Geometry: final body of the model. Coordinates: model frame, mm. A direction names the side the tool comes from. Coordinates: 2 decimals unless noted, no trailing zeros. Order: outer loops, then holes, each group sorted by start corner. A loop starts at its lowest first (then second) coordinate and runs counter-clockwise, first axis right, second up. Notation, with made-up numbers: (22, -10.75) - (73, -10.75) arc R9 cw to (73, -5.75) - close; hole circle Ø2 at (62, 18). An arc over 180 degrees is marked (long way). Use one line per item in the form item = value. Start each with the question number.
```python
from build123d import *

# Parameters (mm, degrees)
CROQUIS1_R              = 1
SALIENTE_EXTRUIR1_DEPTH = 1.6
CROQUIS2_R              = 1
CORTAR_EXTRUIR1_DEPTH   = 10
CROQUIS3_R              = 6
CROQUIS3_W              = 4.6
CROQUIS3_H              = 10
CROQUIS3_W_2            = 6.6
CROQUIS3_H_2            = 6.6
CROQUIS3_W_3            = 5
CROQUIS3_H_3            = 11
CROQUIS3_H_4            = 5
SALIENTE_EXTRUIR2_DEPTH = 2
CROQUIS4_R              = 6
SALIENTE_EXTRUIR3_DEPTH = 4.5
CROQUIS5_W              = 4.6
CROQUIS5_H              = 10
SALIENTE_EXTRUIR4_DEPTH = 1.5
CROQUIS7_R              = 1.122052982
SALIENTE_EXTRUIR5_DEPTH = 1.6
CROQUIS9_R              = 1.125
CORTAR_EXTRUIR2_DEPTH   = 33.479147156


with BuildPart() as part:
    # Croquis1 → Saliente-Extruir1 (new body)
    with BuildSketch(Plane(origin=(0, 0, 0), x_dir=(1, 0, 0), z_dir=(0, 1, 0))):
        Polygon((-18.05, 13.85), (18.05, 13.85), (18.05, 10.8), (28.65, 10.8), (28.65, -10.8), (18.05, -10.8), (18.05, -13.85), (-18.05, -13.85), align=None)
        with Locations(Location((-10.35, -12.3, 0), (0, 0, 270))):
            Circle(CROQUIS1_R, mode=Mode.SUBTRACT)
        with Locations(Location((16.05, -12.3, 0), (0, 0, 270))):
            Circle(CROQUIS1_R, mode=Mode.SUBTRACT)
        with Locations(Location((16.05, 12.3, 0), (0, 0, 270))):
            Circle(CROQUIS1_R, mode=Mode.SUBTRACT)
        with Locations(Location((-10.35, 12.3, 0), (0, 0, 270))):
            Circle(CROQUIS1_R, mode=Mode.SUBTRACT)
    extrude(amount=SALIENTE_EXTRUIR1_DEPTH)

    # Croquis2 → Cortar-Extruir1 (cut)
    with BuildSketch(Plane(origin=(0, 1.6, 0), x_dir=(1, 0, 0), z_dir=(0, 1, 0))):
        with Locations(Location((24.25, 7.25, 0), (0, 0, 270))):
            Circle(CROQUIS2_R)
        with Locations(Location((24.25, -7.25, 0), (0, 0, 270))):
            Circle(CROQUIS2_R)
    extrude(amount=-CORTAR_EXTRUIR1_DEPTH, mode=Mode.SUBTRACT)

    # Croquis3 → Saliente-Extruir2 (add)
    with BuildSketch(Plane(origin=(0, 1.6, 0), x_dir=(1, 0, 0), z_dir=(0, 1, 0))):
        with Locations(Location((-2.979600995, -4.139800498, 0), (0, 0, 270))):
            Circle(CROQUIS3_R)
        with Locations((-14.25, 6.32)):
            Rectangle(CROQUIS3_W, CROQUIS3_H)
        with Locations((-14.25, -6.32)):
            Rectangle(CROQUIS3_W, CROQUIS3_H)
        with Locations((12.6, 6.25)):
            Rectangle(CROQUIS3_W_2, CROQUIS3_H_2)
        with Locations((7.05, -3.35)):
            Rectangle(CROQUIS3_W_3, CROQUIS3_H_3)
        with Locations((-3.063985121, 6.85)):
            Rectangle(CROQUIS3_W_3, CROQUIS3_H_4)
    extrude(amount=SALIENTE_EXTRUIR2_DEPTH)

    # Croquis4 → Saliente-Extruir3 (add)
    with BuildSketch(Plane(origin=(0, 3.6, 0), x_dir=(1, 0, 0), z_dir=(0, 1, 0))):
        with Locations(Location((-2.979600995, -4.139800498, 0), (0, 0, 270))):
            Circle(CROQUIS4_R)
    extrude(amount=SALIENTE_EXTRUIR3_DEPTH)

    # Croquis5 → Saliente-Extruir4 (add)
    with BuildSketch(Plane(origin=(0, 3.6, 0), x_dir=(1, 0, 0), z_dir=(0, 1, 0))):
        with Locations((-14.25, 6.32)):
            Rectangle(CROQUIS5_W, CROQUIS5_H)
        with Locations((-14.25, -6.32)):
            Rectangle(CROQUIS5_W, CROQUIS5_H)
    extrude(amount=SALIENTE_EXTRUIR4_DEPTH)

    # Croquis7 → Saliente-Extruir5 (add)
    with BuildSketch(Plane.XZ):
        with Locations((24.25, -7.25)):
            Circle(CROQUIS7_R)
    extrude(amount=-SALIENTE_EXTRUIR5_DEPTH)

    # Croquis9 → Cortar-Extruir2 (cut, through all)
    with BuildSketch(Plane(origin=(0, 1.6, 0), x_dir=(1, 0, 0), z_dir=(0, 1, 0))):
        with Locations(Location((24.25, 7.35, 0), (0, 0, 270))):
            Circle(CROQUIS9_R)
    extrude(amount=-CORTAR_EXTRUIR2_DEPTH, mode=Mode.SUBTRACT)


solid = part.part
```
(1) Cut plane B-B on z = -12.3. Return the cut outline in (x, y).
(2) Material intervals for L1, parallel to X at y = 0.85, z = -12.3; L2, parallel to X at y = 2.75, z = -4.75; L3, parallel to Z at x = -12, y = 4, sorted ascending. Write a range as from..to.
(3) Contact query for flat-ended pins moving along their axis: pin 1 Ø1.7 at (y, z) = (4, 4) entering from +X; pin 2 Ø1 at (x, y) = (-15, 4) entering from +Z; pin 3 Ø1.6 at (y, z) = (3, -7) entering from -X; pin 4 Ø1.6 at (x, z) = (16.05, 12.3) entering from -Y. Output: stop coordinate, or through.
(4) Cut plane C-C on y = 0.75. Return the cut outline in (x, z) (3 decimals), plus the area to 3 significant figures.
(5) Cut plane D-D on z = -7.35. Return the cut outline in (x, y) (3 decimals).
(6) Set-up query: faces 1 (the flat face through (18.05, 1, -12)), 2 (the flat face through (-14, 5.1, 6)), 3 (the flat face through (-14, 3, -11.32)). Return all of +Z, -Z, +X, -X, +Y, -Y with unobstructed straight access to the full face (end or side cutting, diameter ignored); none if empty.
(7) Draft query along Z for faces 4 (the flat face through (28.65, 1, 0)), 5 (the flat face through (23, 1, -10.8)), 6 (the cylindrical face through (25.365, 0.811, -7.496)). Return one class per face: released by +Z, released by -Z, zero draft, split by the parting line, or undercut.
(8) Cut plane A-A on x = -10.35. Return the cut outline in (y, z).
Check sheet entries:
q1.outline = (-18.05, 0) - (-11.35, 0) - (-11.35, 1.6) - (-18.05, 1.6) - close; (-9.35, 0) - (15.05, 0) - (15.05, 1.6) - (-9.35, 1.6) - close; (17.05, 0) - (18.05, 0) - (18.05, 1.6) - (17.05, 1.6) - close
q2.L1 = -18.05..-11.35, -9.35..15.05, 17.05..18.05
q2.L2 = -16.55..-11.95, -5.56..-0.56, 9.3..15.9
q2.L3 = -11.32..-1.32, 1.32..11.32
q3.pin_1 = 9.55
q3.pin_2 = 11.32
q3.pin_3 = -16.55
q3.pin_4 = through
q4.outline = (-18.05, -13.85) - (18.05, -13.85) - (18.05, -10.8) - (28.65, -10.8) - (28.65, 10.8) - (18.05, 10.8) - (18.05, 13.85) - (-18.05, 13.85) - close; hole circle Ø2 at (-10.35, -12.3); hole circle Ø2 at (-10.35, 12.3); hole circle Ø2 at (16.05, -12.3); hole circle Ø2 at (16.05, 12.3); hole circle Ø2.25 at (24.25, -7.35); hole circle Ø2 at (24.25, 7.25)
q4.area = 1,210 mm^2
q5.outline = (-18.05, 0) - (23.125, 0) - (23.125, 1.6) - (15.9, 1.6) - (15.9, 3.6) - (9.3, 3.6) - (9.3, 1.6) - (-0.564, 1.6) - (-0.564, 3.6) - (-5.564, 3.6) - (-5.564, 1.6) - (-11.95, 1.6) - (-11.95, 5.1) - (-16.55, 5.1) - (-16.55, 1.6) - (-18.05, 1.6) - close; (25.375, 0) - (28.65, 0) - (28.65, 1.6) - (25.375, 1.6) - close
q6.face_1 = -Z, +X, +Y, -Y
q6.face_2 = +Z, -Z, -X, +Y
q6.face_3 = -Z, +X, -X, +Y
q7.face_4 = zero draft
q7.face_5 = released by -Z
q7.face_6 = undercut
q8.outline = (0, -13.85) - (1.6, -13.85) - (1.6, -13.3) - (0, -13.3) - close; (0, -11.3) - (1.6, -11.3) - (1.6, 11.3) - (0, 11.3) - close; (0, 13.3) - (1.6, 13.3) - (1.6, 13.85) - (0, 13.85) - close
